from build123d import *

# Parameters (mm, degrees)
CROQUIS2_R              = 1.5
CROQUIS2_R_2            = 6
SALIENTE_EXTRUIR2_DEPTH = 2.9
CROQUIS4_R              = 2
CORTAR_EXTRUIR1_DEPTH   = 12.5
MATRIZC1_COUNT          = 6
CROQUIS5_R              = 1.5
CORTAR_EXTRUIR2_DEPTH   = 10
CROQUIS6_R              = 14
CORTAR_EXTRUIR3_DEPTH   = 1.5


with BuildPart() as part:
    # Croquis2 → Saliente-Extruir2 (new body)
    with BuildSketch(Plane.XY):
        with BuildLine():
            Line((-10.5, 28.115792599), (-10.5, 37.559952077))
            ThreePointArc((-10.5, 37.559952077), (-19.5, 33.774990748), (-27.277872663, 27.873242778))
            Line((-27.277872663, 27.873242778), (-19.098990638, 23.151163039))
            add(Edge.make_bspline(
                [(-29.598990638, 4.96462956), (-22.416381166, 12.9421037), (-19.098990638, 23.151163039)],
                knots=[0, 0, 0, 1, 1, 1], degree=2))
            Line((-29.598990638, 4.96462956), (-37.777872663, 9.686709299))
            ThreePointArc((-37.777872663, 9.686709299), (-39, 0), (-37.777872663, -9.686709299))
            Line((-37.777872663, -9.686709299), (-29.598990638, -4.96462956))
            add(Edge.make_bspline(
                [(-19.098990638, -23.151163039), (-22.416381166, -12.9421037), (-29.598990638, -4.96462956)],
                knots=[0, 0, 0, 1, 1, 1], degree=2))
            Line((-19.098990638, -23.151163039), (-27.277872663, -27.873242778))
            ThreePointArc((-27.277872663, -27.873242778), (-19.5, -33.774990748), (-10.5, -37.559952077))
            Line((-10.5, -37.559952077), (-10.5, -28.115792599))
            add(Edge.make_bspline(
                [(10.5, -28.115792599), (0, -25.884207401), (-10.5, -28.115792599)],
                knots=[0, 0, 0, 1, 1, 1], degree=2))
            Line((10.5, -28.115792599), (10.5, -37.559952077))
            ThreePointArc((10.5, -37.559952077), (19.5, -33.774990748), (27.277872663, -27.873242778))
            Line((27.277872663, -27.873242778), (19.098990638, -23.151163039))
            add(Edge.make_bspline(
                [(29.598990638, -4.96462956), (22.416381166, -12.9421037), (19.098990638, -23.151163039)],
                knots=[0, 0, 0, 1, 1, 1], degree=2))
            Line((29.598990638, -4.96462956), (37.777872663, -9.686709299))
            ThreePointArc((37.777872663, -9.686709299), (38.693261906, -4.88175), (39, 0))
            ThreePointArc((39, 0), (38.693261906, 4.88175), (37.777872663, 9.686709299))
            Line((37.777872663, 9.686709299), (29.598990638, 4.96462956))
            add(Edge.make_bspline(
                [(19.098990638, 23.151163039), (22.416381166, 12.9421037), (29.598990638, 4.96462956)],
                knots=[0, 0, 0, 1, 1, 1], degree=2))
            Line((19.098990638, 23.151163039), (27.277872663, 27.873242778))
            ThreePointArc((27.277872663, 27.873242778), (19.5, 33.774990748), (10.5, 37.559952077))
            Line((10.5, 37.559952077), (10.5, 28.115792599))
            add(Edge.make_bspline(
                [(-10.5, 28.115792599), (0, 25.884207401), (10.5, 28.115792599)],
                knots=[0, 0, 0, 1, 1, 1], degree=2))
        make_face()
        with Locations((-17.142037335, -29.69087961)):
            Circle(CROQUIS2_R, mode=Mode.SUBTRACT)
        with Locations((-34.28407467, 0)):
            Circle(CROQUIS2_R, mode=Mode.SUBTRACT)
        with Locations((17.142037335, -29.69087961)):
            Circle(CROQUIS2_R, mode=Mode.SUBTRACT)
        with Locations((-17.142037335, 29.69087961)):
            Circle(CROQUIS2_R, mode=Mode.SUBTRACT)
        Circle(CROQUIS2_R_2, mode=Mode.SUBTRACT)
        with Locations((34.28407467, 0)):
            Circle(CROQUIS2_R, mode=Mode.SUBTRACT)
        with Locations((17.142037335, 29.69087961)):
            Circle(CROQUIS2_R, mode=Mode.SUBTRACT)
    extrude(amount=SALIENTE_EXTRUIR2_DEPTH)

    # Croquis4 → Cortar-Extruir1 (cut, symmetric)
    with BuildSketch(Plane(origin=(0, 0, 0), x_dir=(0, 0, -1), z_dir=(1, 0, 0))):
        with Locations((1.75, 34.5)):
            Circle(CROQUIS4_R)
    cortar_extruir1 = extrude(amount=CORTAR_EXTRUIR1_DEPTH, both=True, mode=Mode.SUBTRACT)

    # MatrizC1: Cortar-Extruir1 ×6 about axis
    matrizc1_axis = Axis((0, 0, 0), (0, 0, 1))
    for i in range(1, MATRIZC1_COUNT):
        add(cortar_extruir1.rotate(matrizc1_axis, i * 360 / MATRIZC1_COUNT), mode=Mode.SUBTRACT)

    # Croquis5 → Cortar-Extruir2 (cut)
    with BuildSketch(Plane.XY.offset(2.9)):
        with Locations((11, 0)):
            Circle(CROQUIS5_R)
        with Locations((0, -11)):
            Circle(CROQUIS5_R)
        with Locations((-11, 0)):
            Circle(CROQUIS5_R)
        with Locations((0, 11)):
            Circle(CROQUIS5_R)
    extrude(amount=-CORTAR_EXTRUIR2_DEPTH, mode=Mode.SUBTRACT)

    # Croquis6 → Cortar-Extruir3 (cut)
    with BuildSketch(Plane.XY.offset(2.9)):
        Circle(CROQUIS6_R)
    extrude(amount=-CORTAR_EXTRUIR3_DEPTH, mode=Mode.SUBTRACT)


solid = part.part
Source: CAD feature listing. Evaluate the final solid. Frame: model axes, mm. A direction names the side the tool comes from. Coordinates: 2 decimals unless noted, no trailing zeros. Write each loop counter-clockwise with the first axis right and the second up, starting at its lowest first coordinate (ties: lowest second). Pieces come first, ordered by that corner, then holes. Notation, with made-up numbers: M 24.5,26 L 35.5,26 A34 cw 35.5,65 Z; hole C 72.25,87.5 d4. An arc over 180 degrees is marked long. Use a Markdown table: item, result.
1) Ray query, L1, parallel to Y at x = 0, z = 2.4; L2, parallel to X at y = 30, z = 0.45; L3, parallel to Y at x = 0, z = 1.05. Return the intervals inside material, ascending.
Conclusion:
| item | result |
|---|---|
| L1 | y = -27 to -14, 14 to 27 |
| L2 | x = -24.92 to -18.61, -15.67 to -10.5, 10.5 to 15.67, 18.61 to 24.92 |
| L3 | y = -27 to -12.5, -9.5 to -6, 6 to 9.5, 12.5 to 27 |
2) Mould query, pull axis X, two halves, no side actions, for faces 1 (the cylindrical face through (-24.13, 27.23, 0.25)), 2 (the flat face through (-1, -16, 2.9)), 3 (the cylindrical face through (-19.619, -33.706, 1.43)). Classes: pulls with the +X half, pulls with the -X half, needs draft (parallel to the pull), parting line crosses it, or undercut.
Conclusion:
| item | result |
|---|---|
| face 1 | undercut |
| face 2 | needs draft |
| face 3 | pulls with the -X half |
3) Reachability of faces 4 (the flat face through (33.63, -7.29, 1.43)), 5 (the cylindrical face through (12.932, -5.362, 2.16)), 6 (the cylindrical face through (-11.49, 34.51, 0.25)) from +Z, -Z, +X, -X, +Y, -Y: full face, straight path, thin tool, end or side. Return the list, or none.
Conclusion:
| item | result |
|---|---|
| face 4 | +Z, -Z, -Y |
| face 5 | +Z |
| face 6 | -Z |
4) Section B-B, the plane x = 0. Give the number of separate pieces and of enclosed holes in the cut face, then the cut area to 3 significant figures.
Conclusion:
| item | result |
|---|---|
| separate pieces | 4 |
| enclosed holes | 0 |
| area | 89.4 mm^2 |
5) First-contact query: pin 1 Ø1.8 at (x, y) = (-17.14, -29.69) entering from -Z; pin 2 Ø1 at (x, z) = (-3.5, 2) entering from -Y; pin 3 Ø1.5 at (y, z) = (34, 1.5) entering from -X; pin 4 Ø1.5 at (x, z) = (-27.5, 0.5) entering from +Y. Flat tips, straight axial feed; report the tip coordinate or a pass-through.
Conclusion:
| item | result |
|---|---|
| pin 1 | passes through |
| pin 2 | stops at y = -27.16 |
| pin 3 | stops at x = -20.38 |
| pin 4 | stops at y = 28.38 |
6) Section A-A, the plane x = -11.5. Output: boundary loops of the cut face in (y, z), then the cut area to 3 significant figures.
Conclusion:
| item | result |
|---|---|
| outline | M -37.27,0 L -35.47,0 A2 cw -33.53,0 L -1.41,0 L -1.41,1.4 L -7.98,1.4 L -7.98,2.9 L -37.27,2.9 Z; M 1.41,0 L 33.53,0 A2 cw 35.47,0 L 37.27,0 L 37.27,2.9 L 7.98,2.9 L 7.98,1.4 L 1.41,1.4 Z |
| area | 188 mm^2 |
